```python
from build123d import *

# Parameters (mm, degrees)
BOX001_W                = 46
BOX001_H                = 50
BOX001_DEPTH            = 1
CYLINDER006_R           = 7.5
CYLINDER006_DEPTH       = 25
CYLINDER006_PITCH_ANGLE = 90
CYLINDER005_R           = 5
CYLINDER005_DEPTH       = 46
CYLINDER005_PITCH_ANGLE = 90
CYLINDER004_R           = 4.5
CYLINDER004_DEPTH       = 20
CYLINDER004_ROLL_ANGLE  = 90
CYLINDER003_R           = 1.6
CYLINDER003_DEPTH       = 10
CYLINDER002_R           = 1.6
CYLINDER002_DEPTH       = 10
CYLINDER001_R           = 1.6
CYLINDER001_DEPTH       = 10
CYLINDER_R              = 1.6
CYLINDER_DEPTH          = 10
BOX_W                   = 46
BOX_H                   = 50
BOX_DEPTH               = 10


with BuildPart() as cubo001:
    # Box001 → Box001 (new body)
    with BuildSketch(Plane.XY.offset(9.5)):
        with Locations((23, 25)):
            Rectangle(BOX001_W, BOX001_H)
    extrude(amount=BOX001_DEPTH)


with BuildPart() as cilindro006:
    # Cylinder006 → Cylinder006 (new body)
    with BuildSketch(Plane.XY):
        Circle(CYLINDER006_R)
    extrude(amount=CYLINDER006_DEPTH)


with BuildPart() as cilindro006_1:
    # Cylinder006 pitch: moved
    add(cilindro006.part.rotate(Axis((0, 0, 0), (0, 1, 0)), CYLINDER006_PITCH_ANGLE))


with BuildPart() as cilindro006_2:
    # Cylinder006 placement: moved
    add(cilindro006_1.part.moved(Location((10.5, 28, 10))))


with BuildPart() as cilindro005:
    # Cylinder005 → Cylinder005 (new body)
    with BuildSketch(Plane.XY):
        Circle(CYLINDER005_R)
    extrude(amount=CYLINDER005_DEPTH)


with BuildPart() as cilindro005_1:
    # Cylinder005 pitch: moved
    add(cilindro005.part.rotate(Axis((0, 0, 0), (0, 1, 0)), CYLINDER005_PITCH_ANGLE))


with BuildPart() as cilindro005_2:
    # Cylinder005 placement: moved
    add(cilindro005_1.part.moved(Location((0, 28, 10))))


with BuildPart() as cilindro004:
    # Cylinder004 → Cylinder004 (new body)
    with BuildSketch(Plane.XY):
        Circle(CYLINDER004_R)
    extrude(amount=CYLINDER004_DEPTH)


with BuildPart() as cilindro004_1:
    # Cylinder004 roll: moved
    add(cilindro004.part.rotate(Axis((0, 0, 0), (1, 0, 0)), CYLINDER004_ROLL_ANGLE))


with BuildPart() as cilindro004_2:
    # Cylinder004 placement: moved
    add(cilindro004_1.part.moved(Location((23, 20, 10))))


with BuildPart() as cilindro003:
    # Cylinder003 → Cylinder003 (new body)
    with BuildSketch(Plane(origin=(34, 42, 0), x_dir=(1, 0, 0), z_dir=(0, 0, 1))):
        Circle(CYLINDER003_R)
    extrude(amount=CYLINDER003_DEPTH)


with BuildPart() as cilindro002:
    # Cylinder002 → Cylinder002 (new body)
    with BuildSketch(Plane(origin=(12, 42, 0), x_dir=(1, 0, 0), z_dir=(0, 0, 1))):
        Circle(CYLINDER002_R)
    extrude(amount=CYLINDER002_DEPTH)


with BuildPart() as cilindro001:
    # Cylinder001 → Cylinder001 (new body)
    with BuildSketch(Plane(origin=(34, 10, 0), x_dir=(1, 0, 0), z_dir=(0, 0, 1))):
        Circle(CYLINDER001_R)
    extrude(amount=CYLINDER001_DEPTH)


with BuildPart() as cilindro:
    # Cylinder → Cylinder (new body)
    with BuildSketch(Plane(origin=(12, 10, 0), x_dir=(1, 0, 0), z_dir=(0, 0, 1))):
        Circle(CYLINDER_R)
    extrude(amount=CYLINDER_DEPTH)


with BuildPart() as cut007:
    # Box → Box (new body)
    with BuildSketch(Plane.XY):
        with Locations((23, 25)):
            Rectangle(BOX_W, BOX_H)
    extrude(amount=BOX_DEPTH)

    # Cut: cut Cilindro
    add(cilindro.part, mode=Mode.SUBTRACT)

    # Cut001: cut Cilindro001
    add(cilindro001.part, mode=Mode.SUBTRACT)

    # Cut002: cut Cilindro002
    add(cilindro002.part, mode=Mode.SUBTRACT)

    # Cut003: cut Cilindro003
    add(cilindro003.part, mode=Mode.SUBTRACT)

    # Cut004: cut Cilindro004
    add(cilindro004_2.part, mode=Mode.SUBTRACT)

    # Cut005: cut Cilindro005
    add(cilindro005_2.part, mode=Mode.SUBTRACT)

    # Cut006: cut Cilindro006
    add(cilindro006_2.part, mode=Mode.SUBTRACT)

    # Cut007: cut Cubo001
    add(cubo001.part, mode=Mode.SUBTRACT)


solid = cut007.part
```
Geometry check sheet. Reference: the model listing, model coordinates, mm. A direction names the side the tool comes from. Coordinates: 2 decimals unless noted, no trailing zeros. Order: outer loops, then holes, each group sorted by start corner. A loop starts at its lowest first (then second) coordinate and runs counter-clockwise, first axis right, second up. Notation, with made-up numbers: (7, -0.75) - (43, -0.75) arc R12 cw to (43, 9.25) - close; hole circle Ø8 at (0.5, -35). An arc over 180 degrees is marked (long way). Answer in a Markdown table with one row per item. Add a question column.
1. Section check C-C (z = 6.5). Enter the section's corners in (x, y).
2. Section check D-D (y = 28). Enter the section's corners in (x, z).
3. Access from +Z, -Z, +X, -X, +Y, -Y to the whole of each face (thin tool, end or side, straight path). Record for faces 1 (the face through (10.4, 42.07, 4.68)), 2 (the face through (35.5, 28, 4)), 3 (the face through (22.9, 10.1, 5.5)).
4. Draft check along Y on faces 4 (the face through (23, 42, 9.5)), 5 (the face through (23, 50, 5)), 6 (the face through (10.4, 10.07, 4.68)). Enter one of: +Y half, -Y half, draft (parallel to the pull), parting line (faces both ways), or undercut.
5. Gauge pin test, flat ends, axial feed: pin 1 Ø3 at (x, z) = (24, 8) entering from -Y; pin 2 Ø2.5 at (x, y) = (12, 42) entering from +Z. Record the tip position at first contact, or that the pin passes through.
6. Section check B-B (x = 12). Enter the section's corners in (y, z).
7. Section check A-A (y = 10). Enter the section's corners in (x, z), plus the area to 3 significant figures.
8. Material ranges on L1, parallel to X at y = 42, z = 2.75; L2, parallel to X at y = 34.5, z = 6.75; L3, parallel to Y at x = 11.5, z = 1.25, recorded low to high. Write a range as [from, to].
Data:
| question | item | result |
|---|---|---|
| 1 | outline | (0, 0) - (20.17, 0) - (20.17, 20) - (25.83, 20) - (25.83, 0) - (46, 0) - (46, 24.43) - (35.5, 24.43) - (35.5, 21.37) - (10.5, 21.37) - (10.5, 24.43) - (0, 24.43) - close; (0, 31.57) - (10.5, 31.57) - (10.5, 34.63) - (35.5, 34.63) - (35.5, 31.57) - (46, 31.57) - (46, 50) - (0, 50) - close; hole circle Ø3.2 at (12, 10); hole circle Ø3.2 at (12, 42); hole circle Ø3.2 at (34, 10); hole circle Ø3.2 at (34, 42) |
| 2 | outline | (0, 0) - (46, 0) - (46, 5) - (35.5, 5) - (35.5, 2.5) - (10.5, 2.5) - (10.5, 5) - (0, 5) - close |
| 3 | face 1 | +Z, -Z |
| 3 | face 2 | +Z |
| 3 | face 3 | +Z, -Y |
| 4 | face 4 | draft |
| 4 | face 5 | +Y half |
| 4 | face 6 | undercut |
| 5 | pin 1 | stops at y = 20 |
| 5 | pin 2 | passes through |
| 6 | outline | (0, 0) - (8.4, 0) - (8.4, 9.5) - (0, 9.5) - close; (11.6, 0) - (40.4, 0) - (40.4, 9.5) - (35.48, 9.5) arc R7.5 cw to (20.52, 9.5) - (11.6, 9.5) - close; (43.6, 0) - (50, 0) - (50, 9.5) - (43.6, 9.5) - close |
| 7 | outline | (0, 0) - (10.4, 0) - (10.4, 9.5) - (0, 9.5) - close; (13.6, 0) - (32.4, 0) - (32.4, 9.5) - (27.47, 9.5) arc R4.5 cw to (18.53, 9.5) - (13.6, 9.5) - close; (35.6, 0) - (46, 0) - (46, 9.5) - (35.6, 9.5) - close |
| 7 | area | 349 mm² |
| 8 | L1 | x = [0, 10.4], [13.6, 32.4], [35.6, 46] |
| 8 | L2 | x = [0, 10.5], [35.5, 46] |
| 8 | L3 | y = [0, 8.48], [11.52, 40.48], [43.52, 50] |
